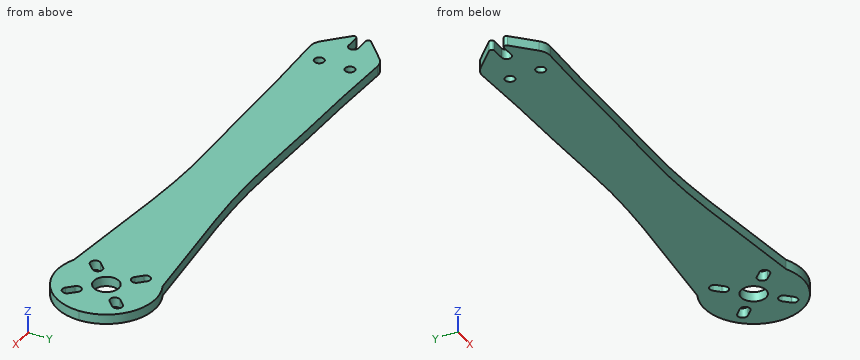
```python
from build123d import *

# Parameters (mm, degrees)
F0_R     = 1.5
F1_DEPTH = 3


with BuildPart() as f1:
    # F0 (on Top) → F1 (new body)
    with BuildSketch(Plane.XY):
        with BuildLine():
            add(Edge.make_bspline(
                [(-6.6800528609, -13.709098941), (-13.6230988968, -12.966112559), (-28.8193966293, -11.35995774), (-60.2323159734, -8.0478026259), (-85.0190153768, -9.5661829277), (-109.9805836112, -9.5257147655), (-126.15485479, -10.2021136613), (-131.7499125902, -10.4552480482)],
                knots=[0, 0, 0, 0, 0.1644519416, 0.3597938043, 0.5352021003, 0.7184076683, 0.848432272, 0.848432272, 0.848432272, 0.848432272], degree=3))
            ThreePointArc((-6.6800528609, -13.709098941), (8.08367781, -12.9312278251), (15.25, 0))
            ThreePointArc((15.25, 0), (8.08367781, 12.9312278251), (-6.6800528609, 13.709098941))
            add(Edge.make_bspline(
                [(-6.6800528609, 13.709098941), (-13.6230988968, 12.966112559), (-28.8193966293, 11.35995774), (-60.2323159734, 8.0478026259), (-85.0190153768, 9.5661829277), (-109.9803350442, 9.5257151685), (-126.1543522734, 10.2020926465), (-131.749284441, 10.4552196292)],
                knots=[0, 0, 0, 0, 0.1644519416, 0.3597938043, 0.5352021003, 0.7184076683, 0.8484274061, 0.8484274061, 0.8484274061, 0.8484274061], degree=3))
            ThreePointArc((-131.749284441, 10.4552196292), (-133.73517656, 10.1403618969), (-135.4364624932, 9.0686674097))
            Line((-135.4364624932, 9.0686674097), (-141.8819995216, 2.8859654139))
            ThreePointArc((-141.8819995216, 2.8859654139), (-142.0716378967, 2.0047030481), (-141.324737254, 1.4999996692))
            Line((-141.324737254, 1.4999996692), (-137.3156530508, 1.4999996692))
            ThreePointArc((-137.3156530508, 1.4999996692), (-135.8156530508, -3.308e-07), (-137.3156530508, -1.5000003308))
            Line((-137.3156530508, -1.5000003308), (-141.3248578726, -1.5000003308))
            ThreePointArc((-141.3248578726, -1.5000003308), (-142.0717522528, -2.0046881347), (-141.8821443687, -2.8859428339))
            Line((-141.8821443687, -2.8859428339), (-135.4372426608, -9.0685515427))
            ThreePointArc((-135.4372426608, -9.0685515427), (-133.7359031159, -10.1403539548), (-131.7499125902, -10.4552480482))
        make_face()
        with Locations((-126.8158406019, -4.75)):
            Circle(F0_R, mode=Mode.SUBTRACT)
        with BuildLine():
            Line((-8.8412747136, -6.7199543701), (-7.019418932, -4.8980985885))
            ThreePointArc((-7.019418932, -4.8980985885), (-4.8980985885, -4.8980985885), (-4.8980985885, -7.019418932))
            Line((-4.8980985885, -7.019418932), (-6.7199543701, -8.8412747136))
            ThreePointArc((-6.7199543701, -8.8412747136), (-8.8412747136, -8.8412747136), (-8.8412747136, -6.7199543701))
        make_face(mode=Mode.SUBTRACT)
        with BuildLine():
            ThreePointArc((4.8980985885, -7.019418932), (4.8980985885, -4.8980985885), (7.019418932, -4.8980985885))
            Line((7.019418932, -4.8980985885), (8.8412747136, -6.7199543701))
            ThreePointArc((8.8412747136, -6.7199543701), (8.8412747136, -8.8412747136), (6.7199543701, -8.8412747136))
            Line((6.7199543701, -8.8412747136), (4.8980985885, -7.019418932))
        make_face(mode=Mode.SUBTRACT)
        with Locations((-126.8158406019, 4.75)):
            Circle(F0_R, mode=Mode.SUBTRACT)
        with BuildLine():
            ThreePointArc((-3.875, 0), (0, 3.875), (3.875, 0))
            ThreePointArc((3.875, 0), (0, -3.875), (-3.875, 0))
        make_face(mode=Mode.SUBTRACT)
        with BuildLine():
            ThreePointArc((-8.8412747136, 6.7199543701), (-8.8412747136, 8.8412747136), (-6.7199543701, 8.8412747136))
            Line((-6.7199543701, 8.8412747136), (-4.8980985885, 7.019418932))
            ThreePointArc((-4.8980985885, 7.019418932), (-4.8980985885, 4.8980985885), (-7.019418932, 4.8980985885))
            Line((-7.019418932, 4.8980985885), (-8.8412747136, 6.7199543701))
        make_face(mode=Mode.SUBTRACT)
        with BuildLine():
            Line((8.8412747136, 6.7199543701), (7.019418932, 4.8980985885))
            ThreePointArc((7.019418932, 4.8980985885), (4.8980985885, 4.8980985885), (4.8980985885, 7.019418932))
            Line((4.8980985885, 7.019418932), (6.7199543701, 8.8412747136))
            ThreePointArc((6.7199543701, 8.8412747136), (8.8412747136, 8.8412747136), (8.8412747136, 6.7199543701))
        make_face(mode=Mode.SUBTRACT)
    extrude(amount=F1_DEPTH)


solid = f1.part
```
Check sheet for the modelled part. Datum: model origin and axes. Units: mm. Give positions to 0.01 mm unless a question says otherwise; leave off trailing zeros. One line per question, with ' | ' between items. Start each with the question number.
1. Cross-section at A-A, the plane z = 2. Give the number of separate pieces and of enclosed holes in the cut face, plus the area to 3 significant figures.
2. Gauge pin test, flat ends, axial feed: pin 1 Ø1.5 at (x, z) = (-139.5, 2) entering from +Y; pin 2 Ø1.8 at (x, y) = (-126.82, 4.75) entering from +Z; pin 3 Ø1.5 at (y, z) = (-4.5, 1) entering from +X; pin 4 Ø3.5 at (x, y) = (-126.82, -4.75) entering from -Z. Record the tip position at first contact, or that the pin passes through.
3. Material ranges on line 1 along X through (y, z) = (-6.5, 0.55); line 2 along Y through (x, z) = (5, 1.1); line 3 along Y through (x, z) = (0, 2.25) (3 decimals), recorded low to high. Write a range as [from, to].
Check result:
1) separate pieces: 1 | enclosed holes: 7 | area: 3,110 mm2
2) pin 1: stops at y = 5.89 | pin 2: passes through | pin 3: stops at x = 14.78 | pin 4: stops at z = 0
3) line 1: x = [-138.11, -8.62], [-4.56, 4.56], [8.62, 13.8] | line 2: y = [-14.41, -7.12], [-4.81, 4.81], [7.12, 14.41] | line 3: y = [-15.25, -3.875], [3.875, 15.25]
